Here's how the part is built. I have some questions about the finished solid (model axes, mm). A direction names the side the tool comes from. Coordinates: 2 decimals unless noted, no trailing zeros. Loops run counter-clockwise (first coordinate to the right, second up) from the corner with the lowest first, then second, coordinate; pieces in that order, holes last. Notation, with made-up numbers: (48, 10) -> (74, 10) arc R22 cw to (74, 45) -> close; hole circle Ø8 at (54.25, -38). An arc over 180 degrees is marked (long way). Use CSV: the item, a comma, the result in double quotes. Start each with the question number.
from build123d import *

# Parameters (mm, degrees)
EXTRUDE_1_DEPTH     = 40
SKETCH_2_R          = 1.65
SKETCH_2_W          = 27
SKETCH_2_H          = 22
CUT_EXTRUDE_2_DEPTH = 10
SKETCH_3_R          = 2
CUT_EXTRUDE_3_DEPTH = 10


with BuildPart() as part:
    # 草图1 → 凸台-拉伸1 (new body)
    with BuildSketch(Plane.XY):
        Polygon((0, 0), (30, 0), (30, -60), (27, -60), (27, -3), (0, -3), align=None)
    extrude(amount=EXTRUDE_1_DEPTH)

    # 草图2 → 切除-拉伸2 (cut)
    with BuildSketch(Plane(origin=(0, 0, 0), x_dir=(1, 0, 0), z_dir=(0, 1, 0))):
        with Locations((7.5, -4.5)):
            Circle(SKETCH_2_R)
        with Locations((19.5, -4.5)):
            Circle(SKETCH_2_R)
        with Locations((19.5, -35.5)):
            Circle(SKETCH_2_R)
        with Locations((7.5, -35.5)):
            Circle(SKETCH_2_R)
        with Locations((13.5, -20)):
            Rectangle(SKETCH_2_W, SKETCH_2_H)
    extrude(amount=-CUT_EXTRUDE_2_DEPTH, mode=Mode.SUBTRACT)

    # 草图3 → 切除-拉伸3 (cut)
    with BuildSketch(Plane(origin=(30, 0, 0), x_dir=(0, 0, -1), z_dir=(1, 0, 0))):
        with Locations((-25, -5)):
            Circle(SKETCH_3_R)
        with Locations((-15, -5)):
            Circle(SKETCH_3_R)
        with Locations((-15, -55)):
            Circle(SKETCH_3_R)
        with Locations((-25, -55)):
            Circle(SKETCH_3_R)
        Polygon((-20.75, -9.5), (-20.75, -2.75), (-19.25, -2.75), (-19.25, -9.5), (-9, -9.5), (-9, -50.5), (-19.25, -50.5), (-19.25, -57.25), (-20.75, -57.25), (-20.75, -50.5), (-31, -50.5), (-31, -9.5), align=None)
    extrude(amount=-CUT_EXTRUDE_3_DEPTH, mode=Mode.SUBTRACT)


solid = part.part
1) I want a section at D-D, the plane x = 7.5. Please give me the cut outline in (y, z).
2) I want a section at C-C, the plane z = 4.5. Please give me the cut outline in (x, y).
3) Which directions (+Z, -Z, +X, -X, +Y, -Y) give clear straight access to the entire face, cutting with the end or side of a thin tool? Please do faces 1 (the face through (29, -30, 31)), 2 (the face through (7.285, -1.479, 33.864)), 3 (the face through (14, -3, 4)).
4) I want a section at B-B, the plane y = -5. Please give me the cut outline in (x, z), plus the area to 3 significant figures.
5) I want a section at A-A, the plane z = 20. Please give me the cut outline in (x, y).
6) Please list where these lines run through material, in increasing order: L1, parallel to X at y = -0.7, z = 4.5; L2, parallel to Y at x = 28.05, z = 25; L3, parallel to Z at x = 7.5, y = -1.95. Write a range as [from, to].
7) For P1, Ø8, axis at x = 21, z = 32, coming from the -Y side; P2, Ø1.5, axis at x = 12, z = 28.5, coming from the +Y side, each with a flat end and sliding along its axis, tell me the tip position at first contact or that it passes through.
8) Thinking about a two-plate mould opening in X: for faces 4 (the face through (29, -6, 20.75)), 5 (the face through (18.19, -1.48, 5.5)), 6 (the face through (27, -30, 34)), 7 (the face through (30, -30, 6)), which applies, pulls with the +X half, pulls with the -X half, needs draft (parallel to the pull), parting line crosses it, or undercut?
Return value:
1,outline,"(-3, 0) -> (0, 0) -> (0, 2.85) -> (-3, 2.85) -> close; (-3, 6.15) -> (0, 6.15) -> (0, 9) -> (-3, 9) -> close; (-3, 31) -> (0, 31) -> (0, 33.85) -> (-3, 33.85) -> close; (-3, 37.15) -> (0, 37.15) -> (0, 40) -> (-3, 40) -> close"
2,outline,"(0, -3) -> (5.85, -3) -> (5.85, 0) -> (0, 0) -> close; (9.15, -3) -> (17.85, -3) -> (17.85, 0) -> (9.15, 0) -> close; (21.15, -3) -> (27, -3) -> (27, -60) -> (30, -60) -> (30, 0) -> (21.15, 0) -> close"
3,face 1,"+X, -X"
3,face 2,"+Y, -Y"
3,face 3,"+Z, -Z, -X, -Y"
4,outline,"(27, 0) -> (30, 0) -> (30, 13) -> (27, 13) -> close; (27, 17) -> (30, 17) -> (30, 19.25) -> (27, 19.25) -> close; (27, 20.75) -> (30, 20.75) -> (30, 23) -> (27, 23) -> close; (27, 27) -> (30, 27) -> (30, 40) -> (27, 40) -> close"
4,area,"91.5 mm²"
5,outline,"(27, -60) -> (30, -60) -> (30, -57.25) -> (27, -57.25) -> close; (27, -2.75) -> (30, -2.75) -> (30, 0) -> (27, 0) -> close"
6,L1,"x = [0, 5.85], [9.15, 17.85], [21.15, 30]"
6,L2,"y = [-60, -57], [-53, -50.5], [-9.5, -7], [-3, 0]"
6,L3,"z = [0, 2.85], [6.15, 9], [31, 33.85], [37.15, 40]"
7,P1,"stops at y = -3"
7,P2,"passes through"
8,face 4,"needs draft"
8,face 5,"undercut"
8,face 6,"pulls with the -X half"
8,face 7,"pulls with the +X half"
